from build123d import *

# Parameters (mm, degrees)
F1_DEPTH  = 90
F2_R      = 11
F3_DEPTH  = 25
F5_DEPTH  = 25
F6_R      = 1.75
F7_DEPTH  = 25
F9_R      = 3
F10_DEPTH = 25
F12_R     = 3
F13_DEPTH = 25
F14_SIZE  = 2
F15_R     = 1
F17_DEPTH = 1.5
F19_DEPTH = 1.5


with BuildPart() as f1:
    # F0 (on Top) → F1 (new body)
    with BuildSketch(Plane.XY):
        Polygon((70, 89), (61, 89), (11, 30), (11, 21), (19, 21), (19, 30), (19, 33.3303359461), (19, 37.1198922439), (56.1865319967, 81), (61, 81), (70, 81), align=None)
    extrude(amount=F1_DEPTH)

    # F2 (on face) → F3 (cut)
    with BuildSketch(Plane(origin=(-8.3947500418, 7.1141949507, 0), x_dir=(-0.6465216954, -0.7628956006, 0), z_dir=(-0.7628956006, 0.6465216954, 0))):
        with Locations((-68.6670692686, 67.5)):
            Circle(F2_R)
        with Locations((-68.6670692686, 22.5)):
            Circle(F2_R)
    extrude(amount=-F3_DEPTH, mode=Mode.SUBTRACT)

    # F4 (on face) → F5 (cut)
    with BuildSketch(Plane.XZ.offset(-21)):
        with BuildLine():
            ThreePointArc((16.75, 75), (16.2374368671, 76.2374368671), (15, 76.75))
            Line((15, 76.75), (15, 73.25))
            ThreePointArc((15, 73.25), (16.2374368671, 73.7625631329), (16.75, 75))
        make_face()
        with BuildLine():
            ThreePointArc((16.75, 15), (16.2374368671, 16.2374368671), (15, 16.75))
            Line((15, 16.75), (15, 13.25))
            ThreePointArc((15, 13.25), (16.2374368671, 13.7625631329), (16.75, 15))
        make_face()
        with BuildLine():
            Line((15, 13.25), (15, 16.75))
            ThreePointArc((15, 16.75), (13.25, 15), (15, 13.25))
        make_face()
        with BuildLine():
            Line((15, 73.25), (15, 76.75))
            ThreePointArc((15, 76.75), (13.25, 75), (15, 73.25))
        make_face()
    extrude(amount=-F5_DEPTH, mode=Mode.SUBTRACT)

    # F6 (on face) → F7 (cut)
    with BuildSketch(Plane.YZ.offset(70)):
        with Locations((85, 75)):
            Circle(F6_R)
        with Locations((85, 15)):
            Circle(F6_R)
    extrude(amount=-F7_DEPTH, mode=Mode.SUBTRACT)

    # F9 (on offset) → F10 (cut)
    with BuildSketch(Plane.YZ.offset(65)):
        with Locations((85, 75)):
            Circle(F9_R)
        with Locations((85, 15)):
            Circle(F9_R)
    extrude(amount=-F10_DEPTH, mode=Mode.SUBTRACT)

    # F12 (on offset) → F13 (cut)
    with BuildSketch(Plane.XZ.offset(-26)):
        with Locations((15, 75)):
            Circle(F12_R)
        with Locations((15, 15)):
            Circle(F12_R)
    extrude(amount=-F13_DEPTH, mode=Mode.SUBTRACT)

    # F14
    f14_edges = [f1.edges().sort_by_distance(p)[0] for p in [
        (70, 81, 45),
        (70, 89, 45),
        (19, 21, 45),
        (11, 21, 45),
    ]]
    chamfer(f14_edges, length=F14_SIZE)

    # F15
    f15_edges = [f1.edges().sort_by_distance(p)[0] for p in [
        (61, 89, 45),
        (11, 30, 45),
    ]]
    fillet(f15_edges, radius=F15_R)

    # F16 (on face) → F17 (join)
    with BuildSketch(Plane.XY.offset(90)):
        Polygon((19, 37.1198922439), (19, 30.0599461219), (61, 30.0599461219), (61, 81), (56.1865319967, 81), align=None)
    extrude(amount=-F17_DEPTH)

    # F18 (on face) → F19 (join)
    with BuildSketch(Plane.XY):
        Polygon((61, 30), (61, 81), (56.1865319967, 81), (19, 37.1198922439), (19, 30), align=None)
    extrude(amount=F19_DEPTH)


solid = f1.part
Part model, mm, in its own coordinate system. A direction names the side the tool comes from. Round coordinates to 2 decimals unless told otherwise and drop trailing zeros. Write each loop counter-clockwise with the first axis right and the second up, starting at its lowest first coordinate (ties: lowest second). Pieces come first, ordered by that corner, then holes. Notation, with made-up numbers: M -33.5,85.25 L -4.5,85.25 A16 ccw -4.5,102.25 Z; hole C -35.75,38 d6. An arc over 180 degrees is marked long. Return JSON: item names as keys, results as strings. Group by question number.
(1) Drill centre lines: probe 1 along Z at (x, y) = (67, 85); probe 2 along Z at (x, y) = (59, 85); probe 3 along Z at (x, y) = (51.5, 72). Where is each one in solid material? Low to high.
(2) Saw through at D-D on x = 34.5. Count the separate pieces of the cut face and the enclosed holes in it, then the cut area to 3 significant figures.
(3) Pin check, flat tips, straight feed: pin 1 Ø1.5 at (y, z) = (60.5, 47.5) entering from -X; pin 2 Ø5 at (x, z) = (15, 15) entering from -Y; pin 3 Ø5 at (y, z) = (85, 15) entering from -X; pin 4 Ø2 at (y, z) = (64.5, 32) entering from -X. Stop position of each tip, or through.
(4) Two-plate mould, pull along X, no slides. Class faces 1 (the face through (17.86, 30.68, 15.9)), 2 (the face through (17, 26, 15)), 3 (the face through (38.11, 60.84, 11.76)), 4 (the face through (61, 82, 75)): +X half, -X half, draft (parallel to the pull), parting line (faces both ways), or undercut.
(5) Saw through at C-C on x = 27. Write the cut outline in (y, z).
(6) Which spindle directions (+Z, -Z, +X, -X, +Y, -Y) get a long thin tool onto all of the face, cutting with end or side? Do faces 5 (the face through (61, 82, 15)), 6 (the face through (70, 85, 44)), 7 (the face through (17.86, 30.68, 75.9)), 8 (the face through (44, 50, 1.5)), 9 (the face through (67.535, 86.669, 15.526)). Say none if no direction does.
(7) Saw through at B-B on y = 85. Write the cut outline in (x, z), then the cut area to 3 significant figures.
(8) Saw through at A-A on z = 49.5. Write the cut outline in (x, y), then the cut area to 3 significant figures.
Returned:
{
 "1": {"probe 1": "0 to 13.25, 16.75 to 73.25, 76.75 to 90", "probe 2": "0 to 12, 18 to 72, 78 to 90", "probe 3": "0 to 1.5, 88.5 to 90"},
 "2": {"separate pieces": "3", "enclosed holes": "0", "area": "187 mm²"},
 "3": {"pin 1": "x = 36.21", "pin 2": "y = 21", "pin 3": "x = 65", "pin 4": "x = 39.4"},
 "4": {"face 1": "undercut", "face 2": "undercut", "face 3": "parting line", "face 4": "draft"},
 "5": {"outline": "M 30,0 L 48.88,0 L 48.88,90 L 30.06,90 L 30.06,88.5 L 46.56,88.5 L 46.56,1.5 L 30,1.5 Z"},
 "6": {"face 5": "-X", "face 6": "+Z, -Z, +X, +Y, -Y", "face 7": "+Y", "face 8": "+X, -Y", "face 9": "+X, -X"},
 "7": {"outline": "M 57.61,0 L 70,0 L 70,13.25 L 65,13.25 L 65,12 L 57.61,12 Z; M 57.61,18 L 65,18 L 65,16.75 L 70,16.75 L 70,73.25 L 65,73.25 L 65,72 L 57.61,72 Z; M 57.61,78 L 65,78 L 65,76.75 L 70,76.75 L 70,90 L 57.61,90 Z", "area": "991 mm²"},
 "8": {"outline": "M 11,23 L 13,21 L 17,21 L 19,23 L 19,37.12 L 56.19,81 L 68,81 L 70,83 L 70,87 L 68,89 L 61.46,89 A1 ccw 60.7,88.65 L 11.24,30.28 A1 ccw 11,29.63 Z", "area": "285 mm²"}
}
